from build123d import *

# Parameters (mm, degrees)
SKETCH_1_W      = 46
SKETCH_1_H      = 20
SKETCH_1_R      = 3.5
SKETCH_1_R_2    = 3
EXTRUDE_1_DEPTH = 1.5
SKETCH_2_R      = 5
SKETCH_2_R_2    = 3.5
EXTRUDE_2_DEPTH = 0.5
SKETCH_3_W      = 46
SKETCH_3_H      = 20
SKETCH_3_W_2    = 43.5
SKETCH_3_H_2    = 16.5
EXTRUDE_3_DEPTH = 20
SKETCH_4_R      = 1.75
EXTRUDE_4_DEPTH = 3
FILLET_1_R      = 2
EXTRUDE_5_DEPTH = 2
FILLET_2_R      = 2


with BuildPart() as part:
    # Эскиз1 → Бобышка-Вытянуть1 (new body)
    with BuildSketch(Plane.XY):
        with Locations((23, 10)):
            Rectangle(SKETCH_1_W, SKETCH_1_H)
        with Locations((7.5, 12)):
            Circle(SKETCH_1_R, mode=Mode.SUBTRACT)
        with Locations((38.5, 10)):
            Circle(SKETCH_1_R_2, mode=Mode.SUBTRACT)
    extrude(amount=EXTRUDE_1_DEPTH)

    # Эскиз2 → Бобышка-Вытянуть2 (add)
    with BuildSketch(Plane(origin=(0, 0, 0), x_dir=(-1, 0, 0), z_dir=(0, 0, -1))):
        with Locations((-7.5, 12)):
            Circle(SKETCH_2_R)
        with Locations((-7.5, 12)):
            Circle(SKETCH_2_R_2, mode=Mode.SUBTRACT)
    extrude(amount=EXTRUDE_2_DEPTH)

    # Эскиз3 → Бобышка-Вытянуть3 (add)
    with BuildSketch(Plane(origin=(0, 0, 0), x_dir=(-1, 0, 0), z_dir=(0, 0, -1))):
        with Locations((-23, 10)):
            Rectangle(SKETCH_3_W, SKETCH_3_H)
        with Locations((-22.75, 10.25)):
            Rectangle(SKETCH_3_W_2, SKETCH_3_H_2, mode=Mode.SUBTRACT)
    extrude(amount=EXTRUDE_3_DEPTH)

    # Эскиз4 → Бобышка-Вытянуть4 (add)
    with BuildSketch(Plane.XZ):
        with BuildLine():
            Line((0, 1.5), (-4, 1.5))
            ThreePointArc((-4, 1.5), (-8, -2.5), (-4, -6.5))
            Line((-4, -6.5), (0, -6.5))
            Line((0, -6.5), (0, 1.5))
        make_face()
        with Locations((-4, -2.5)):
            Circle(SKETCH_4_R, mode=Mode.SUBTRACT)
        with BuildLine():
            Line((50, 1.5), (46, 1.5))
            Line((46, 1.5), (46, -6.5))
            Line((46, -6.5), (50, -6.5))
            ThreePointArc((50, -6.5), (54, -2.5), (50, 1.5))
        make_face()
        with Locations((50, -2.5)):
            Circle(SKETCH_4_R, mode=Mode.SUBTRACT)
    extrude(amount=-EXTRUDE_4_DEPTH)

    # Скругление1
    fillet_1_edges = [part.edges().sort_by_distance(p)[0] for p in [
        (0, 1.5, -6.5),
        (46, 1.5, -6.5),
    ]]
    fillet(fillet_1_edges, radius=FILLET_1_R)

    # Эскиз5 → Бобышка-Вытянуть5 (add)
    with BuildSketch(Plane.XZ):
        Polygon((41, -20), (35, -20), (35, -27), (36.5, -27), (36.5, -30), (35, -30), (35, -32), (41, -32), (41, -30), (39.5, -30), (39.5, -27), (41, -27), align=None)
        Polygon((11, -20), (5, -20), (5, -27), (6.5, -27), (6.5, -30), (5, -30), (5, -32), (11, -32), (11, -30), (9.5, -30), (9.5, -27), (11, -27), align=None)
    extrude(amount=-EXTRUDE_5_DEPTH)

    # Скругление2
    fillet_2_edges = [part.edges().sort_by_distance(p)[0] for p in [
        (41, 1, -20),
        (35, 1, -20),
        (11, 1, -20),
        (5, 1, -20),
    ]]
    fillet(fillet_2_edges, radius=FILLET_2_R)


solid = part.part
Here's how the part is built. I have some questions about the finished solid (model axes, mm). A direction names the side the tool comes from. Give positions to 0.01 mm unless a question says otherwise; leave off trailing zeros. Write each loop counter-clockwise with the first axis right and the second up, starting at its lowest first coordinate (ties: lowest second). Pieces come first, ordered by that corner, then holes. Notation, with made-up numbers: (-22, 15) -> (-11, 15) arc R10 ccw to (-11, 28) -> close; hole circle Ø2 at (80, -17). An arc over 180 degrees is marked (long way). Use one line per item in the form item = value. Start each with the question number.
1. Thinking about a two-plate mould opening in Z: for faces 1 (the face through (41, 1, -31)), 2 (the face through (51.617, 1.479, -3.17)), 3 (the face through (4.4, 1.01, -20.57)), 4 (the face through (36, 1, -27)), which applies, +Z half, -Z half, draft (parallel to the pull), parting line (faces both ways), or undercut?
2. On a 3-axis mill with a long thin cutter (end or side, diameter ignored), from which of +Z, -Z, +X, -X, +Y, -Y can I reach the whole of each face in a straight line? I mean faces 5 (the face through (10, 1, -27)), 6 (the face through (5, 1, -24)), 7 (the face through (22, 10, 0)), 8 (the face through (6, 1, -30)), 9 (the face through (40, 1, -27)). Say none if no direction works.
3. Imagine slicing it at D-D on z = -16.5. List the corners of the cut face in (x, y) for me, plus the area to 3 significant figures.
4. If I drill on L1, parallel to Y at x = 9, z = -5.5; L2, parallel to X at y = 1, z = -28.5; L3, parallel to Z at x = -4, y = 2.2, over which ranges is the centre line in solid material (lowest first)?
5. Imagine slicing it at C-C on x = 38.5. List the corners of the cut face in (y, z) for me.
6. Imagine slicing it at A-A on z = -2.5. List the corners of the cut face in (x, y) for me, plus the area to 3 significant figures.
7. Will these pins go through, and if not, where does the flat tip stop? pin 1 Ø0.6 at (y, z) = (1, -31) entering from -X; pin 2 Ø10 at (x, y) = (29.5, 11) entering from -Z; pin 3 Ø0.6 at (y, z) = (1, -28.5) entering from -X.
8. Imagine slicing it at B-B on y = 10. List the corners of the cut face in (x, z) for me.
Entries:
q1.face_1 = draft
q1.face_2 = undercut
q1.face_3 = -Z half
q1.face_4 = undercut
q2.face_5 = +Y, -Y
q2.face_6 = -Z, -X, +Y, -Y
q2.face_7 = -Z
q2.face_8 = -X, +Y, -Y
q2.face_9 = +X, +Y, -Y
q3.outline = (0, 0) -> (46, 0) -> (46, 20) -> (0, 20) -> close; hole (1, 2) -> (44.5, 2) -> (44.5, 18.5) -> (1, 18.5) -> close
q3.area = 202 mm²
q4.L1 = 0 to 2, 18.5 to 20
q4.L2 = 6.5 to 9.5, 36.5 to 39.5
q4.L3 = -6.5 to -4.25, -0.75 to 1.5
q5.outline = (0, -32) -> (2, -32) -> (2, 0) -> (7, 0) -> (7, 1.5) -> (0, 1.5) -> close; (13, 0) -> (18.5, 0) -> (18.5, -20) -> (20, -20) -> (20, 1.5) -> (13, 1.5) -> close
q6.outline = (-8, 0) -> (-5.75, 0) -> (-5.75, 3) -> (-8, 3) -> close; (-2.25, 0) -> (48.25, 0) -> (48.25, 3) -> (46, 3) -> (46, 20) -> (0, 20) -> (0, 3) -> (-2.25, 3) -> close; (51.75, 0) -> (54, 0) -> (54, 3) -> (51.75, 3) -> close; hole (1, 2) -> (44.5, 2) -> (44.5, 18.5) -> (1, 18.5) -> close
q6.area = 229 mm²
q7.pin_1 = 5
q7.pin_2 = 0
q7.pin_3 = 6.5
q8.outline = (0, -20) -> (1, -20) -> (1, 0) -> (2.92, 0) -> (2.92, -0.5) -> (4.63, -0.5) -> (4.63, 1.5) -> (0, 1.5) -> close; (10.37, -0.5) -> (12.08, -0.5) -> (12.08, 0) -> (35.5, 0) -> (35.5, 1.5) -> (10.37, 1.5) -> close; (41.5, 0) -> (44.5, 0) -> (44.5, -20) -> (46, -20) -> (46, 1.5) -> (41.5, 1.5) -> close
